Check sheet for the drawn part. Datum: minimum x, y, z corner. Units: mm. A direction names the side the tool comes from. Round coordinates to 2 decimals unless told otherwise and drop trailing zeros. Write each loop counter-clockwise with the first axis right and the second up, starting at its lowest first coordinate (ties: lowest second). Pieces come first, ordered by that corner, then holes. Notation, with made-up numbers: (64, 11) - (97, 11) arc R15 cw to (97, 39) - close; hole circle Ø1 at (-29, -37.5). An arc over 180 degrees is marked (long way). Answer as a JSON object with one key per item and string values.
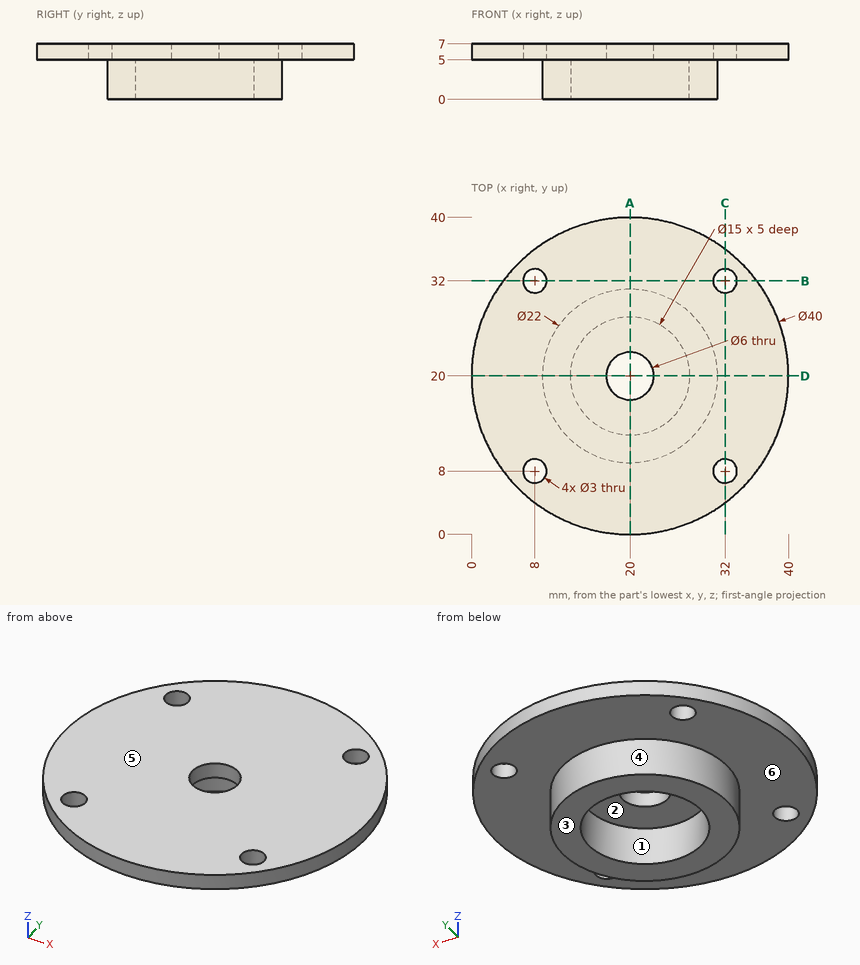
Q1. Section check B-B, the plane y = 32. Record the cut outline in (x, z), then the cut area to 3 significant figures.
Geometry check:
{"outline": "(4, 5) - (6.5, 5) - (6.5, 7) - (4, 7) - close; (9.5, 5) - (30.5, 5) - (30.5, 7) - (9.5, 7) - close; (33.5, 5) - (36, 5) - (36, 7) - (33.5, 7) - close", "area": "52.0 mm2"}
Q2. Release check for a two-part mould opening along Y. For the marked faces 1, 2, 3 and 4 record: released by +Y, released by -Y, zero draft, split by the parting line, or undercut.
Geometry check:
{"face 1": "undercut", "face 2": "undercut", "face 3": "zero draft", "face 4": "split by the parting line"}
Q3. Gauge pin test, flat ends, axial feed: P1, Ø3.5, axis at x = 32, y = 8, coming from the -Z side; P2, Ø5, axis at x = 32, y = 32, coming from the +Z side; P3, Ø2.5, axis at x = 8, y = 32, coming from the +Z side; P4, Ø1, axis at x = 23, z = 3.5, coming from the +Y side. Record the tip position at first contact, or that the pin passes through.
Geometry check:
{"P1": "stops at z = 5", "P2": "stops at z = 7", "P3": "passes through", "P4": "stops at y = 30.71"}
Q4. Material ranges on line 1 along Y through (x, z) = (8, 6.15); line 2 along Z through (x, y) = (9, 12); line 3 along X through (y, z) = (9, 6), recorded low to high. Write a range as [from, to].
Geometry check:
{"line 1": "y = [4, 6.5], [9.5, 30.5], [33.5, 36]", "line 2": "z = [5, 7]", "line 3": "x = [3.3, 6.88], [9.12, 30.88], [33.12, 36.7]"}
Q5. Section check A-A, the plane x = 20. Record the cut outline in (y, z), then the cut area to 3 significant figures.
Geometry check:
{"outline": "(0, 5) - (9, 5) - (9, 0) - (12.5, 0) - (12.5, 5) - (17, 5) - (17, 7) - (0, 7) - close; (23, 5) - (27.5, 5) - (27.5, 0) - (31, 0) - (31, 5) - (40, 5) - (40, 7) - (23, 7) - close", "area": "103 mm2"}
Q6. Set-up check for the marked faces 5 and 6: record each of +Z, -Z, +X, -X, +Y, -Y from which the full face is reachable in a straight line by a thin tool's end or side.
Geometry check:
{"face 5": "+Z, +X, -X, +Y, -Y", "face 6": "-Z"}
